```python
from build123d import *

# Parameters (mm, degrees)
CUT_EXTRUDE1_DEPTH = 33.258177258
FILLET1_R          = 6


with BuildPart() as part:
    # Sketch2 → Revolve1 (revolve)
    with BuildSketch(Plane.XY, mode=Mode.PRIVATE) as revolve1_sk:
        Polygon((8, 2.3), (8, 5.3), (12.5, 5.3), (16.5, 3), (22.5, 3), (22.5, 0), (15.698988524, 0), (11.698988524, 2.3), align=None)
    revolve(revolve1_sk.sketch.rotate(Axis((0, 0, 0), (0, 1, 0)), 90), axis=Axis((0, 0, 0), (0, 1, 0)))

    # Sketch3 → Cut-Extrude1 (cut, through all)
    with BuildSketch(Plane(origin=(0, 0, 0), x_dir=(1, 0, 0), z_dir=(0, 1, 0))):
        with BuildLine():
            Line((-5.1, 21.914378841), (-5.1, 6.163602842))
            ThreePointArc((-5.1, 6.163602842), (0, 8), (5.1, 6.163602842))
            Line((5.1, 6.163602842), (5.1, 21.914378841))
            ThreePointArc((5.1, 21.914378841), (0, 22.5), (-5.1, 21.914378841))
        make_face()
    extrude(amount=CUT_EXTRUDE1_DEPTH, mode=Mode.SUBTRACT)

    # Fillet1
    fillet1_edges = [part.edges().sort_by_distance(p)[0] for p in [
        (0, 0, 15.698988524),
        (0, 3, 16.5),
        (0, 5.3, 12.5),
    ]]
    fillet(fillet1_edges, radius=FILLET1_R)


solid = part.part
```
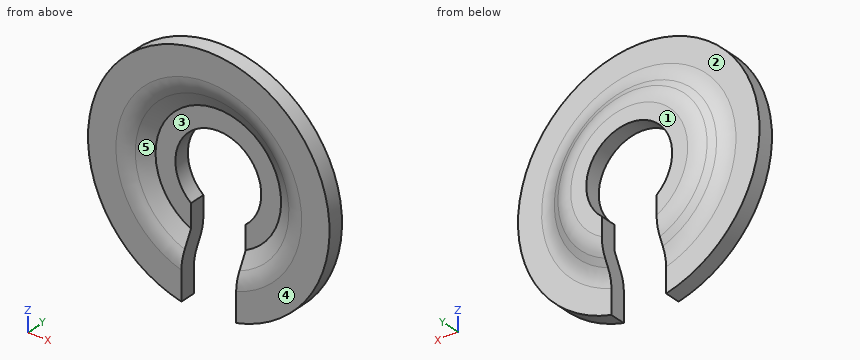
Could you check a few things on this model? Use its own coordinates, in mm. Face numbers are marked on the shaded views. A direction names the side the tool comes from. Coordinates: 2 decimals unless noted, no trailing zeros. Loops run counter-clockwise (first coordinate to the right, second up) from the corner with the lowest first, then second, coordinate; pieces in that order, holes last.
1) Will these pins go through, and if not, where does the flat tip stop? pin 1 Ø1.5 at (y, z) = (2, 6.5) entering from -X; pin 2 Ø2 at (x, z) = (-16.5, 14.5) entering from +Y; pin 3 Ø18.5 at (x, z) = (0, 0) entering from +Y; pin 4 Ø1 at (y, z) = (4, 5.5) entering from +X.
Reported:
pin 1: stops at x = -21.75
pin 2: stops at y = 3
pin 3: stops at y = 5.3
pin 4: stops at x = 14.72
2) Please list where these lines run through material, in increasing order: line 1 along Y through (x, z) = (18.5, 12); line 2 along X through (y, z) = (3.8, 0); line 3 along X through (y, z) = (4.1, 5) (3 decimals).
Reported:
line 1: y = 0 to 3
line 2: x = -15.11 to -8, 8 to 15.11
line 3: x = -13.703 to -6.245, 6.245 to 13.703
3) Imagine slicing it at B-B (x = 0). List the corners of the cut face in (y, z) for me.
Reported:
outline: (0, 17.3) arc R6 ccw to (0.8, 14.31) - (2.3, 11.7) - (2.3, 8) - (5.3, 8) - (5.3, 10.9) arc R6 ccw to (4.5, 13.89) - (3.8, 15.11) arc R6 cw to (3, 18.1) - (3, 22.5) - (0, 22.5) - close
4) Imagine slicing it at C-C (y = 1.55). List the corners of the cut face in (x, z) for me, and give its area (3 significant figures).
Reported:
outline: (-5.1, -21.91) - (-5.1, -11.96) arc R13 cw (long way) to (5.1, -11.96) - (5.1, -21.91) arc R22.5 ccw (long way) to start
area: 961 mm2
5) Imagine slicing it at D-D (x = -19). List the corners of the cut face in (y, z) for me, and give its area (3 significant figures).
Reported:
outline: (0, -12.05) - (3, -12.05) - (3, 12.05) - (0, 12.05) - close
area: 72.3 mm2
6) Which directions (+Z, -Z, +X, -X, +Y, -Y) give clear straight access to the entire face, cutting with the end or side of a thin tool? Please do the marked faces 1, 2 and 3.
Reported:
face 1: +Z, -Z, +X, -X, +Y
face 2: +Y
face 3: -Y
7) Thinking about a two-plate mould opening in Z: for the marked faces 4 and 5, which applies, released by +Z, released by -Z, zero draft, split by the parting line, or undercut?
Reported:
face 4: zero draft
face 5: undercut
8) Imagine slicing it at A-A (z = 0). List the corners of the cut face in (x, y) for me, and give its area (3 significant figures).
Reported:
outline: (-22.5, 0) - (-17.3, 0) arc R6 ccw to (-14.31, 0.8) - (-11.7, 2.3) - (-8, 2.3) - (-8, 5.3) - (-10.9, 5.3) arc R6 ccw to (-13.89, 4.5) - (-15.11, 3.8) arc R6 cw to (-18.1, 3) - (-22.5, 3) - close; (8, 2.3) - (11.7, 2.3) - (14.31, 0.8) arc R6 ccw to (17.3, 0) - (22.5, 0) - (22.5, 3) - (18.1, 3) arc R6 cw to (15.11, 3.8) - (13.89, 4.5) arc R6 ccw to (10.9, 5.3) - (8, 5.3) - close
area: 90.2 mm2
